```python
from build123d import *

# Parameters (mm, degrees)
SKETCH1_W               = 60
SKETCH1_H               = 33
BOSS_EXTRUDE1_DEPTH     = 10
SKETCH2_W               = 4.2
SKETCH2_H               = 11
CUT_EXTRUDE1_DEPTH      = 5.8
BOSS_EXTRUDE2_START     = -45.4
BOSS_EXTRUDE2_DEPTH     = 55.8
SKETCH4_W               = 33
SKETCH4_H               = 2.2
CUT_EXTRUDE2_DEPTH      = 1
CUT_EXTRUDE2_DEPTH_BACK = 61
FILLET1_R               = 2
SKETCH7_W               = 20.8
SKETCH7_H               = 17
CUT_EXTRUDE4_DEPTH      = 16
FILLET2_R               = 2
BOSS_EXTRUDE4_START     = -7.8
SKETCH5_W               = 60
SKETCH5_H               = 5
BOSS_EXTRUDE4_DEPTH     = 55
SKETCH8_W               = 50
SKETCH8_H               = 50
CUT_EXTRUDE5_DEPTH      = 52.15
FILLET3_R               = 10
FILLET4_R               = 5
FILLET6_R               = 5


with BuildPart() as part:
    # Sketch1 → Boss-Extrude1 (new body)
    with BuildSketch(Plane(origin=(0, 0, 0), x_dir=(1, 0, 0), z_dir=(0, 1, 0))):
        with Locations((30, 16.5)):
            Rectangle(SKETCH1_W, SKETCH1_H)
    extrude(amount=BOSS_EXTRUDE1_DEPTH)

    # Sketch2 → Cut-Extrude1 (cut)
    with BuildSketch(Plane(origin=(0, 10, 0), x_dir=(1, 0, 0), z_dir=(0, 1, 0))):
        with Locations((12.5, 23)):
            Rectangle(SKETCH2_W, SKETCH2_H)
        with Locations((47.5, 23)):
            Rectangle(SKETCH2_W, SKETCH2_H)
    extrude(amount=-CUT_EXTRUDE1_DEPTH, mode=Mode.SUBTRACT)

    # Sketch3 → Boss-Extrude2 (add)
    with BuildSketch(Plane.ZY.offset(-14.6).offset(BOSS_EXTRUDE2_START)):
        Polygon((-28.5, 5.85), (-25.1, 8.5), (-25.1, 10), (-28.5, 10), align=None)
    extrude(amount=BOSS_EXTRUDE2_DEPTH)

    # Sketch4 → Cut-Extrude2 (cut, two sides)
    with BuildSketch(Plane(origin=(60, 0, 0), x_dir=(0, 0, -1), z_dir=(1, 0, 0))) as cut_extrude2_sk:
        with Locations((16.5, 1.1)):
            Rectangle(SKETCH4_W, SKETCH4_H)
    extrude(amount=CUT_EXTRUDE2_DEPTH, mode=Mode.SUBTRACT)
    extrude(cut_extrude2_sk.sketch, amount=-CUT_EXTRUDE2_DEPTH_BACK, mode=Mode.SUBTRACT)

    # Fillet1
    fillet1_edges = [part.edges().sort_by_distance(p)[0] for p in [
        (12.5, 10, -17.5),
        (47.5, 10, -17.5),
    ]]
    fillet(fillet1_edges, radius=FILLET1_R)

    # Sketch7 → Cut-Extrude4 (cut)
    with BuildSketch(Plane(origin=(0, 10, 0), x_dir=(1, 0, 0), z_dir=(0, 1, 0))):
        with Locations((30, 19.5)):
            Rectangle(SKETCH7_W, SKETCH7_H)
    extrude(amount=-CUT_EXTRUDE4_DEPTH, mode=Mode.SUBTRACT)

    # Fillet2
    fillet2_edges = [part.edges().sort_by_distance(p)[0] for p in [
        (19.6, 6.1, -11),
        (19.6, 6.1, -28),
        (40.4, 6.1, -28),
        (40.4, 6.1, -11),
    ]]
    fillet(fillet2_edges, radius=FILLET2_R)

    # Sketch5 → Boss-Extrude4 (add)
    with BuildSketch(Plane(origin=(0, 10, 0), x_dir=(1, 0, 0), z_dir=(0, 1, 0)).offset(BOSS_EXTRUDE4_START)):
        with Locations((30, 2.5)):
            Rectangle(SKETCH5_W, SKETCH5_H)
    extrude(amount=-BOSS_EXTRUDE4_DEPTH)

    # Sketch8 → Cut-Extrude5 (cut)
    with BuildSketch(Plane(origin=(0, 0, -5), x_dir=(-1, 0, 0), z_dir=(0, 0, -1))):
        with Locations((-30, -22.8)):
            Rectangle(SKETCH8_W, SKETCH8_H)
    extrude(amount=-CUT_EXTRUDE5_DEPTH, mode=Mode.SUBTRACT)

    # Fillet3
    fillet3_edges = [part.edges().sort_by_distance(p)[0] for p in [
        (57.5, 2.2, -5),
        (2.5, 2.2, -5),
        (55, -47.8, -2.5),
        (55, 2.2, -2.5),
        (5, 2.2, -2.5),
        (5, -47.8, -2.5),
    ]]
    fillet(fillet3_edges, radius=FILLET3_R)

    # Fillet4
    fillet4_edges = [part.edges().sort_by_distance(p)[0] for p in [
        (60, -52.8, -2.5),
        (0, -52.8, -2.5),
    ]]
    fillet(fillet4_edges, radius=FILLET4_R)

    # Fillet6
    fillet6_edges = [part.edges().sort_by_distance(p)[0] for p in [
        (0, 6.1, -33),
        (60, 6.1, -33),
    ]]
    fillet(fillet6_edges, radius=FILLET6_R)


solid = part.part
```
Part model, mm, in its own coordinate system. A direction names the side the tool comes from. Coordinates: 2 decimals unless noted, no trailing zeros. Write each loop counter-clockwise with the first axis right and the second up, starting at its lowest first coordinate (ties: lowest second). Pieces come first, ordered by that corner, then holes.
Item 1: Which spindle directions (+Z, -Z, +X, -X, +Y, -Y) get a long thin tool onto all of the face, cutting with end or side? Do faces 4 (the face through (30, -47.8, -3)), 5 (the face through (12, 5, -28.5)), 6 (the face through (19.6, 6, -19)), 7 (the face through (12, 6, -17.5)). Say none if no direction does.
Item 2: Slice it at B-B (y = -25.5). Write the cut outline in (x, z).
Item 3: Mould opens along Z. For faces 1 (the face through (5, -23, -3)), 2 (the face through (47.53, 9.43, -16.9)), 3 (the face through (58, 6, -32)) say: released by +Z, released by -Z, zero draft, split by the parting line, or undercut.
Item 4: Pin check, flat tips, straight feed: pin 1 (16.5 mm diameter, centred on x = 37, z = -19, fed in from -Y); pin 2 (6 mm diameter, centred on x = 51.5, y = -46, fed in from -Z); pin 3 (12 mm diameter, centred on x = 12, y = -36.5, fed in from -Z). Stop position of each tip, or through.
Item 5: Slice it at C-C (z = -3.5). Write the cut outline in (x, y).
Item 6: Probe line 1 (Y direction, x = 38, z = -3.5); line 2 (X direction, y = 5.5, z = -26.5); line 3 (Y direction, x = 52, z = -22). List the from-to ranges inside material, lowest first.
Item 7: Slice it at A-A (x = 42). Write the cut outline in (y, z).
Item 8: Slice it at D-D (x = 30.5). Write the cut outline in (y, z), and give its area (3 significant figures).
Results found:
1. face 4: +Z, -Z
1. face 5: none
1. face 6: +Y, -Y
1. face 7: +Y
2. outline: (0, -5) - (5, -5) - (5, 0) - (0, 0) - close; (55, -5) - (60, -5) - (60, 0) - (55, 0) - close
3. face 1: zero draft
3. face 2: undercut
3. face 3: released by -Z
4. pin 1: stops at y = 2.2
4. pin 2: stops at z = -5
4. pin 3: passes through
5. outline: (0, -47.8) arc R5 ccw to (5, -52.8) - (55, -52.8) arc R5 ccw to (60, -47.8) - (60, 10) - (0, 10) - close; hole (5, -37.8) arc R10 ccw to (15, -47.8) - (45, -47.8) arc R10 ccw to (55, -37.8) - (55, -7.8) arc R10 ccw to (45, 2.2) - (15, 2.2) arc R10 ccw to (5, -7.8) - close
6. line 1: y = -52.8 to -47.8, 2.2 to 10
6. line 2: x = 0 to 10.4, 14.6 to 19.66, 40.34 to 45.4, 49.6 to 60
6. line 3: y = 2.2 to 10
7. outline: (-52.8, -5) - (-47.8, -5) - (-47.8, 0) - (-52.8, 0) - close; (2.2, -33) - (10, -33) - (10, 0) - (2.2, 0) - close
8. outline: (-52.8, -5) - (-47.8, -5) - (-47.8, 0) - (-52.8, 0) - close; (2.2, -33) - (10, -33) - (10, -28) - (2.2, -28) - close; (2.2, -11) - (10, -11) - (10, 0) - (2.2, 0) - close
8. area: 150 mm2
